Model file for the job. Use its own axes, mm. A direction names the side the tool comes from. Coordinates: 2 decimals unless noted, no trailing zeros. Order: outer loops, then holes, each group sorted by start corner. A loop starts at its lowest first (then second) coordinate and runs counter-clockwise, first axis right, second up.
Autodesk Inventor part; units mm, degrees
ref_plane "YZ Plane" through (0, 0, 0) normal (1, 0, 0) x (0, 1, 0)
ref_plane "XZ Plane" through (0, 0, 0) normal (0, 1, 0) x (-1, 0, 0)
ref_plane "XY Plane" through (0, 0, 0) normal (0, 0, 1) x (1, 0, 0)
sketch "Sketch1" plane through (0, 0, 0) normal (0, 0, 1) x (1, 0, 0)
  line L0 (-101.6, -273.05) -> (-101.6, 6.35)
  line L1 (0, -273.05) -> (0, 6.35)
  line L2 (0, -6.35) -> (-101.6, -6.35)
  line L3 (0, -260.35) -> (-101.6, -260.35)
  point P0 (0, 0)
extrude "Extrusion1" add sketch "Sketch1" against normal blind 6.35
sketch "Sketch2" plane through (-101.6, -260.35, 0) normal (0, -1, 0) x (1, 0, 0)
  line L0 (0, 0) -> (0, -6.35)
  line L1 (101.6, 0) -> (101.6, -6.35)
  line L2 (38.1, 0) -> (63.5, 0)
  line L3 (63.5, 0) -> (63.5, -6.35)
  line L4 (63.5, -6.35) -> (38.1, -6.35)
  line L5 (38.1, -6.35) -> (38.1, 0)
  dimension "d2" = 25.4
  dimension "d3" = 38.1
  dimension "d4" = 38.1
extrude "Extrusion2" add sketch "Sketch2" along normal blind 6.35
ref_plane "Work Plane1" through (-101.6, -133.35, -6.35) normal (0, -1, 0) x (1, 0, 0)
mirror "Mirror1" about plane through (-101.6, -133.35, -6.35) normal (0, -1, 0) of "Extrusion2"
sketch "Sketch3" plane through (0, -260.35, 0) normal (1, 0, 0) x (0, 0, -1)
  line L0 (0, 0) -> (6.35, 0)
  line L1 (0, 254) -> (6.35, 254)
  line L2 (0, 139.7) -> (6.35, 139.7)
  line L3 (6.35, 139.7) -> (6.35, 114.3)
  line L4 (6.35, 114.3) -> (0, 114.3)
  line L5 (0, 114.3) -> (0, 139.7)
  point P0 (0, 260.35)
  dimension "d7" = 25.4
  dimension "d8" = 6.35
  dimension "d9" = 114.3
  dimension "d10" = 114.3
extrude "Extrusion3" add sketch "Sketch3" along normal blind 6.35
ref_plane "Work Plane2" through (-50.8, -260.35, 0) normal (1, 0, 0) x (0, 0, -1)
mirror "Mirror2" about plane through (-50.8, -260.35, 0) normal (1, 0, 0) of "Extrusion3"
sketch "Sketch4" plane through (0, 0, 0) normal (0, 0, 1) x (1, 0, 0)
  line L0 (0, -6.35) -> (0, -120.65)
  line L1 (-38.1, -6.35) -> (0, -6.35)
  line L2 (-25.4, -50.8) -> (-50.8, -50.8)
  line L3 (-50.8, -50.8) -> (-50.8, -76.2)
  line L4 (-50.8, -76.2) -> (-25.4, -76.2)
  line L5 (-25.4, -76.2) -> (-25.4, -50.8)
  point P0 (0, 0)
  dimension "d13" = 25.4
  dimension "d14" = 25.4
  dimension "d15" = 25.4
  dimension "d16" = 44.45
extrude "Extrusion4" cut sketch "Sketch4" against normal through all
sketch "Sketch5" plane through (0, 0, 0) normal (0, 0, 1) x (1, 0, 0)
  line L0 (-101.6, -6.35) -> (-63.5, -6.35)
  line L1 (-101.6, -120.65) -> (-101.6, -6.35)
  line L2 (0, -260.35) -> (-38.1, -260.35)
  circle A0 centre (-83.82, -19.05) radius 3.9687
  circle A1 centre (-83.82, -57.15) radius 3.9687
  circle A2 centre (-83.82, -95.25) radius 3.9687
  circle A3 centre (-83.82, -133.35) radius 3.9687
  circle A4 centre (-83.82, -171.45) radius 3.9687
  circle A5 centre (-83.82, -209.55) radius 3.9687
  circle A6 centre (-83.82, -247.65) radius 3.9687
  circle A7 centre (-45.72, -19.05) radius 3.9687
  circle A8 centre (-45.72, -95.25) radius 3.9687
  circle A9 centre (-45.72, -133.35) radius 3.9687
  circle A10 centre (-45.72, -171.45) radius 3.9687
  circle A11 centre (-45.72, -209.55) radius 3.9687
  circle A12 centre (-45.72, -247.65) radius 3.9687
  point P0 (0, 0)
  dimension "d19" = 7.9375
  dimension "d20" = 17.78
  dimension "d21" = 12.7
  dimension "d24" = 38.1
  dimension "d31" = 38.1
extrude "Extrusion5" cut sketch "Sketch5" against normal through all
sketch "Sketch6" plane through (0, 0, -6.35) normal (0, 0, -1) x (-1, 0, 0)
  line L0 (0, -146.05) -> (0, -260.35)
  line L1 (0, -260.35) -> (38.1, -260.35)
  circle A0 centre (12.7, -247.65) radius 6.35
  point P0 (0, 0)
  dimension "d38" = 12.7
  dimension "d39" = 12.7
  dimension "d40" = 12.7
extrude "Extrusion6" cut sketch "Sketch6" against normal through all
equation "\"d3\" = d4"
equation "\"d9\" = d10"
properties part number "baseBoxLongSide01"
Q1. Cut at C-C, the plane x = -12.7. List the corners of the cut face in (y, z), plus the area to 3 significant figures.
Established:
outline: (-260.35, -6.35) - (-254, -6.35) - (-254, 0) - (-260.35, 0) - close; (-241.3, -6.35) - (-6.35, -6.35) - (-6.35, 0) - (-241.3, 0) - close
area: 1,530 mm2
Q2. Probe line 1 (X direction, y = -134.5, z = -4.5); line 2 (X direction, y = -96, z = -5.5); line 3 (X direction, y = -214.5, z = -3.75). List the from-to ranges inside material, lowest first.
Established:
line 1: x = -107.95 to -87.62, -80.02 to -49.52, -41.92 to 6.35
line 2: x = -101.6 to -87.72, -79.92 to -49.62, -41.82 to 0
line 3: x = -101.6 to 0
Q3. Mould opens along Y. For faces 5 (the face through (-86.969, -135.765, -3.131)), 6 (the face through (-82, -260.35, -3)), 7 (the face through (-38.1, -3, -3)) say: pulls with the +Y half, pulls with the -Y half, needs draft (parallel to the pull), parting line crosses it, or undercut.
Established:
face 5: undercut
face 6: pulls with the -Y half
face 7: needs draft
Q4. Drop flat-ended pins along their axis: P1, Ø1.9, axis at x = -75, z = -3, coming from the +Y side; P2, Ø3, axis at y = -4, z = -2, coming from the -X side; P3, Ø3, axis at x = -24, z = -2.5, coming from the -Y side. Give the stop position or say it passes through.
Established:
P1: stops at y = -6.35
P2: stops at x = -63.5
P3: stops at y = -260.35
Q5. Cut at A-A, the plane y = -57.15. List the corners of the cut face in (x, z), plus the area to 3 significant figures.
Established:
outline: (-101.6, -6.35) - (-87.79, -6.35) - (-87.79, 0) - (-101.6, 0) - close; (-79.85, -6.35) - (-50.8, -6.35) - (-50.8, 0) - (-79.85, 0) - close; (-25.4, -6.35) - (0, -6.35) - (0, 0) - (-25.4, 0) - close
area: 433 mm2
Q6. Cut at B-B, the plane x = -83.82. Count the separate pieces of the cut face and the enclosed holes in it, plus the area to 3 significant figures.
Established:
separate pieces: 8
enclosed holes: 0
area: 1,260 mm2
Q7. Which spindle directions (+Z, -Z, +X, -X, +Y, -Y) get a long thin tool onto all of the face, cutting with end or side? Do faces 1 (the face through (-63.5, -3, -3)), 2 (the face through (-38, -76.2, -3)), 3 (the face through (0, -204, -3)), 4 (the face through (0, -64, -3)). Say none if no direction does.
Established:
face 1: +Z, -Z, -X, +Y
face 2: +Z, -Z
face 3: +Z, -Z, +X, -Y
face 4: +Z, -Z, +X, +Y
